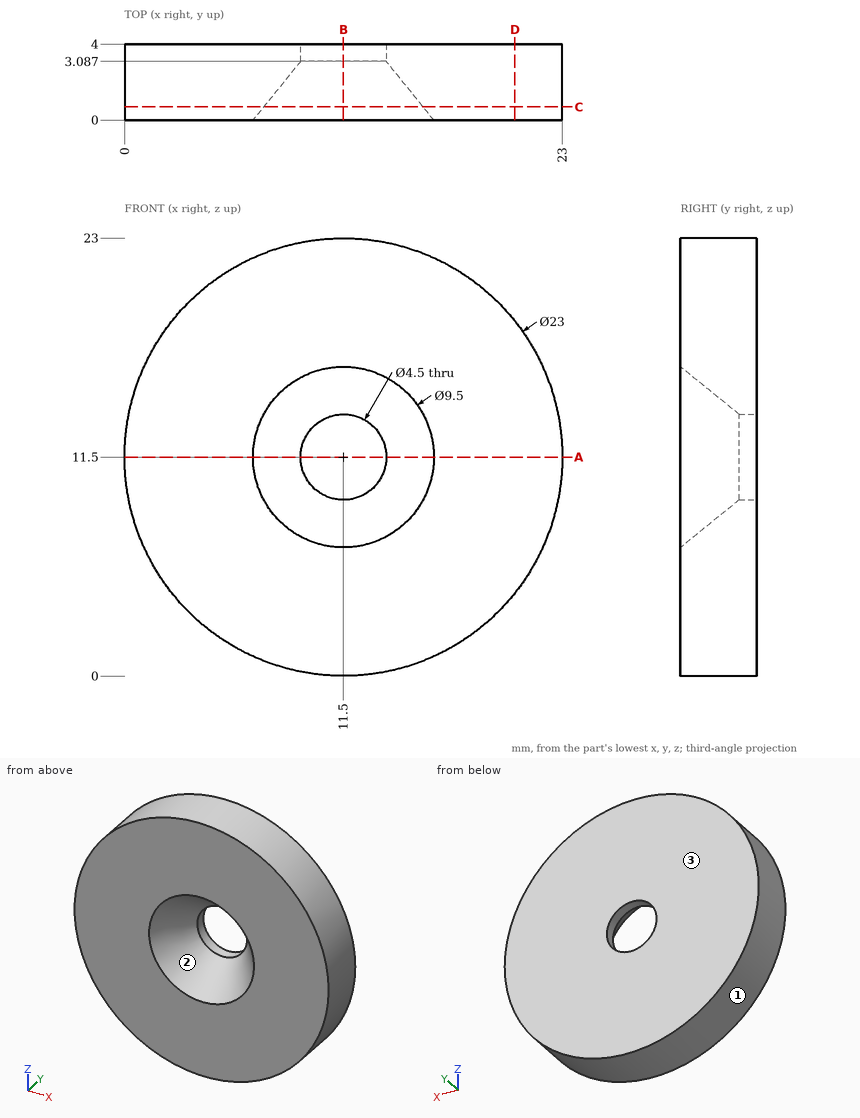
Could you check a few things on this drawing? It's one solid part, dimensions in mm from its lowest x, y, z. Coordinates: 2 decimals unless noted, no trailing zeros. Write each loop counter-clockwise with the first axis right and the second up, starting at its lowest first coordinate (ties: lowest second). Pieces come first, ordered by that corner, then holes.
Q1. Imagine slicing it at C-C, the plane y = 0.7. List the corners of the cut face in (x, z) for me.
Results found:
outline: circle Ø23 at (11.5, 11.5); hole circle Ø8.37 at (11.5, 11.5)
Q2. Imagine slicing it at A-A, the plane z = 11.5. List the corners of the cut face in (x, y) for me, plus the area to 3 significant figures.
Results found:
outline: (0, 0) - (6.75, 0) - (9.25, 3.09) - (9.25, 4) - (0, 4) - close; (13.75, 3.09) - (16.25, 0) - (23, 0) - (23, 4) - (13.75, 4) - close
area: 66.3 mm2
Q3. For P1, Ø1, axis at x = 6, y = 3.5, coming from the +Z side; P2, Ø1, axis at x = 8, z = 13.5, coming from the -Y side, each with a flat end and sliding along its axis, tell me the tip position at first contact or that it passes through.
Results found:
P1: stops at z = 21.86
P2: stops at y = 0.27
Q4. Please list where these lines run through material, in increasing order: L1, parallel to Z at x = 11.5, y = 3.75; L2, parallel to X at y = 2.3, z = 11.75.
Results found:
L1: z = 0 to 9.25, 13.75 to 23
L2: x = 0 to 8.62, 14.38 to 23
Q5. Imagine slicing it at D-D, the plane x = 20.5. List the corners of the cut face in (y, z) for me, plus the area to 3 significant figures.
Results found:
outline: (0, 4.34) - (4, 4.34) - (4, 18.66) - (0, 18.66) - close
area: 57.3 mm2
Q6. If we mould it in two halves opening along Z, with no side actions, what happens to the marked faces 1, 2 and 3? For each: +Z half, -Z half, draft (parallel to the pull), parting line (faces both ways), or undercut.
Results found:
face 1: parting line
face 2: undercut
face 3: draft
Q7. Imagine slicing it at B-B, the plane x = 11.5. List the corners of the cut face in (y, z) for me.
Results found:
outline: (0, 0) - (4, 0) - (4, 9.25) - (3.09, 9.25) - (0, 6.75) - close; (0, 16.25) - (3.09, 13.75) - (4, 13.75) - (4, 23) - (0, 23) - close
